```python
from build123d import *

# Parameters (mm, degrees)
BOSS_EXTRUDE1_DEPTH = 30
CUT_EXTRUDE1_DEPTH  = 20
CHAMFER1_SIZE       = 10
SKETCH4_W           = 20
SKETCH4_H           = 20
CUT_EXTRUDE2_DEPTH  = 41.358334189


with BuildPart() as part:
    # Sketch1 → Boss-Extrude1 (new body)
    with BuildSketch(Plane(origin=(0, 0, 0), x_dir=(1, 0, 0), z_dir=(0, 1, 0))):
        with BuildLine():
            Line((-65.495262312, 61.728199509), (-51.064892932, 53.913448014))
            Line((-51.064892932, 53.913448014), (-15.510423608, 31.112009379))
            Line((-15.510423608, 31.112009379), (17.288542893, 31.112009379))
            Line((17.288542893, 31.112009379), (50.510402672, 53.128986682))
            Line((50.510402672, 53.128986682), (65.676291813, 61.535556337))
            ThreePointArc((65.676291813, 61.535556337), (55.986333501, 70.466520143), (45.096073772, 77.886739118))
            Line((45.096073772, 77.886739118), (41, 61.886739118))
            Line((41, 61.886739118), (-41, 61.886739118))
            Line((-41, 61.886739118), (-45.096073772, 77.886739118))
            ThreePointArc((-45.096073772, 77.886739118), (-55.882783617, 70.548667565), (-65.495262312, 61.728199509))
        make_face()
    extrude(amount=BOSS_EXTRUDE1_DEPTH)

    # Sketch3 → Cut-Extrude1 (cut)
    with BuildSketch(Plane(origin=(0, 30, 0), x_dir=(1, 0, 0), z_dir=(0, 1, 0))):
        Polygon((41, 61.886739118), (41, 39.992019881), (77.260525415, 39.992019881), (80.602533751, 99.084803638), (39.738886371, 90.425963859), align=None)
    cut_extrude1 = extrude(amount=-CUT_EXTRUDE1_DEPTH, mode=Mode.SUBTRACT)

    # Mirror1: Cut-Extrude1 across plane
    add(cut_extrude1.mirror(Plane(origin=(0, 0, 0), x_dir=(0, 0, 1), z_dir=(1, 0, 0))), mode=Mode.SUBTRACT)

    # Chamfer1
    chamfer1_edges = [part.edges().sort_by_distance(p)[0] for p in [
        (41, 30, -54.356469192),
        (-41, 30, -54.672735052),
    ]]
    chamfer(chamfer1_edges, length=CHAMFER1_SIZE)

    # Sketch4 → Cut-Extrude2 (cut)
    with BuildSketch(Plane(origin=(0, 0, -61.886739118), x_dir=(-1, 0, 0), z_dir=(0, 0, -1))):
        with Locations((0, 10)):
            Rectangle(SKETCH4_W, SKETCH4_H)
    extrude(amount=-CUT_EXTRUDE2_DEPTH, mode=Mode.SUBTRACT)


solid = part.part
```
Input: part model. Units: mm. Frame: model coordinates. A direction names the side the tool comes from. Round coordinates to 2 decimals unless told otherwise and drop trailing zeros. Write each loop counter-clockwise with the first axis right and the second up, starting at its lowest first coordinate (ties: lowest second). Pieces come first, ordered by that corner, then holes. Notation, with made-up numbers: M -22.5,57.5 L -14.5,57.5 A18 cw -14.5,66.5 Z; hole C -15.5,87.25 d6. An arc over 180 degrees is marked long. Write each question's results on one line, items separated by ' | '.
Q1. Line query: line 1 along X through (y, z) = (14.5, -47.5); line 2 along Z through (x, y) = (31, 10.5); line 3 along Z through (x, y) = (16.5, 23). Output: solid intervals per line, ascending.
Results:
line 1: x = -41 to -10, 10 to 41 | line 2: z = -61.89 to -40.2 | line 3: z = -61.89 to -31.11
Q2. Section query C-C (x = -6.5). Return loops of the section in (y, z), and give its area (3 significant figures).
Results:
outline: M 20,-61.89 L 30,-61.89 L 30,-31.11 L 20,-31.11 Z | area: 308 mm^2
Q3. Section query A-A (y = 12). Return loops of the section in (x, z).
Results:
outline: M -41,-61.89 L -10,-61.89 L -10,-31.11 L -15.51,-31.11 L -41,-47.46 Z; M 10,-61.89 L 41,-61.89 L 41,-46.83 L 17.29,-31.11 L 10,-31.11 Z
Q4. Access query for faces 1 (the face through (-41, 15, -55)), 2 (the face through (1, 21, -61.887)), 3 (the face through (50, 10, -63)). Directions: +Z, -Z, +X, -X, +Y, -Y. A direction counts if a zero-diameter tool reaches every point of the face in a straight line with its end or side. Return the directions, or none.
Results:
face 1: +Z, -Z, -X, +Y | face 2: -Z, +Y, -Y | face 3: +Z, -Z, +X, +Y
Q5. Pin query (flat end, axial travel): P1, Ø6, axis at y = 10.5, z = -42, coming from the +X side; P2, Ø2, axis at y = 4.5, z = -62, coming from the -X side; P3, Ø15, axis at x = -9.5, y = 18, coming from the -Z side; P4, Ø12, axis at x = 2.5, z = -69.5, coming from the -Y side. Return the tip coordinate at first contact, or that it passes through.
Results:
P1: stops at x = 38.24 | P2: stops at x = -65.5 | P3: stops at z = -61.89 | P4: passes through
Q6. Section query B-B (z = -70). Return loops of the section in (x, y).
Results:
outline: M -56.57,0 L -43.08,0 L -43.08,10 L -56.57,10 Z; M 43.08,0 L 56.57,0 L 56.57,10 L 43.08,10 Z
Q7. Draft query along X for faces 4 (the face through (-36, 25, -54)), 5 (the face through (-50, 10, -63)), 6 (the face through (10, 10, -47)), 7 (the face through (56.13, 4.93, -70.35)). Return one class per face: released by +X, released by -X, zero draft, split by the parting line, or undercut.
Results:
face 4: released by -X | face 5: zero draft | face 6: undercut | face 7: released by +X
Q8. Section query D-D (z = -56.5). Return loops of the section in (x, y).
Results:
outline: M -55.84,0 L -10,0 L -10,20 L 10,20 L 10,0 L 56.59,0 L 56.59,10 L 41,10 L 41,20 L 31,30 L -31,30 L -41,20 L -41,10 L -55.84,10 Z
